Build history of the part. All positions in model axes, mm. Face numbers are marked on the shaded views. A direction names the side the tool comes from. Give positions to 0.01 mm unless a question says otherwise; leave off trailing zeros. Write each loop counter-clockwise with the first axis right and the second up, starting at its lowest first coordinate (ties: lowest second). Pieces come first, ordered by that corner, then holes. Notation, with made-up numbers: M -33.75,40.5 L -5.75,40.5 A21 cw -5.75,47.5 Z; hole C 2,32.25 d11. An arc over 180 degrees is marked long. One line per item, written item: value. Start each with the question number.
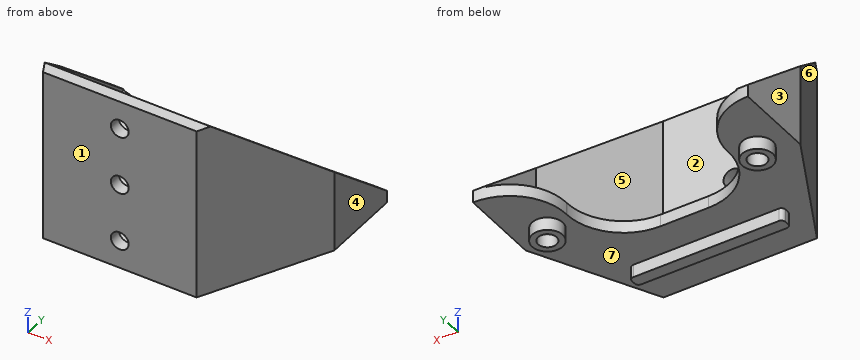
from build123d import *

# Parameters (mm, degrees)
F4_DEPTH       = 21.4
F5_DEPTH       = 1.5
F1_R           = 1.9
F1_W           = 19
F1_H           = 1.5
F6_DEPTH       = 1.6
F8_DEPTH       = 17.001
F8_DEPTH_BACK  = 17.001
F9_R           = 1.15
F10_DEPTH      = 21.401
F10_DEPTH_BACK = 1.601
F11_R          = 1.1
F12_DEPTH      = 1.5
F13_T1_DEPTH   = 1.5
F13_T3_DEPTH   = 36.5
F14_R          = 0.5


# Not quite as in the source:
# - a fillet or chamfer that OpenCascade refuses, or shapes differently, is made with other operations: its cross-section is extruded or revolved along the edge and cut away or added


with BuildPart() as f4:
    # F3 (on face) → F4 (new body)
    with BuildSketch(Plane.XY):
        Polygon((-15.5, 10), (-17, 10), (-17, 0), (-9.5, -14.7), (0, -14.7), (9.5, -14.7), (17, 0), (17, 10), (15.5, 10), (15.5, 0.3605454095), (8.5813543829, -13.2), (0, -13.2), (-8.5813543829, -13.2), (-15.5, 0.3605454095), align=None)
    extrude(amount=F4_DEPTH)

    # F2 (on Top) → F5 (join)
    with BuildSketch(Plane.XY):
        Polygon((-17, 0), (-9.5, -14.7), (0, -14.7), (9.5, -14.7), (17, 0), (17, 10), (10, 10), (10, -4.1), (0, -4.1), (-10, -4.1), (-10, 10), (-17, 10), align=None)
    extrude(amount=F5_DEPTH)

    # F1 (on Top) → F6 (join)
    with BuildSketch(Plane.XY):
        with Locations((-13, 2)):
            Circle(F1_R)
        with Locations((13, 2)):
            Circle(F1_R)
        with Locations((0, -8.95)):
            Rectangle(F1_W, F1_H)
    extrude(amount=-F6_DEPTH)

    # F7 (on Right) → F8 (cut, two sides)
    with BuildSketch(Plane.YZ) as f8_sk:
        Polygon((-13.2, 21.4), (10, 1.5), (10, 21.4), align=None)
    extrude(amount=-F8_DEPTH, mode=Mode.SUBTRACT)
    extrude(f8_sk.sketch, amount=F8_DEPTH_BACK, mode=Mode.SUBTRACT)

    # F9 (on Top) → F10 (cut, two sides)
    with BuildSketch(Plane.XY) as f10_sk:
        with Locations((13, 2)):
            Circle(F9_R)
        with Locations((-13, 2)):
            Circle(F9_R)
    extrude(amount=F10_DEPTH, mode=Mode.SUBTRACT)
    extrude(f10_sk.sketch, amount=-F10_DEPTH_BACK, mode=Mode.SUBTRACT)

    # F11 (on face) → F12 (cut, through all)
    with BuildSketch(Plane.XZ.offset(14.7)):
        with Locations((0, 3.475)):
            Circle(F11_R)
        with Locations((0, 17.925)):
            Circle(F11_R)
        with Locations((0, 10.7)):
            Circle(F11_R)
    extrude(amount=-F12_DEPTH, mode=Mode.SUBTRACT)

    # F13: fillet of radius 7 on 4 edges, made by hand

    # F13_s2 → F13_t1 (join)
    with BuildSketch(Plane.XY):
        with BuildLine():
            ThreePointArc((3, -4.1), (7.9497474683, -2.0497474683), (10, 2.9))
            Line((10, 2.9), (10, -4.1))
            Line((10, -4.1), (3, -4.1))
        make_face()
        with BuildLine():
            ThreePointArc((-10, 2.9), (-7.9497474683, -2.0497474683), (-3, -4.1))
            Line((-3, -4.1), (-10, -4.1))
            Line((-10, -4.1), (-10, 2.9))
        make_face()
    extrude(amount=F13_T1_DEPTH)

    # F13_s4 → F13_t3 (cut)
    with BuildSketch(Plane.XY.offset(-17.5)):
        with BuildLine():
            ThreePointArc((-17, 10), (-12.0502525317, 7.9497474683), (-10, 3))
            Line((-10, 3), (-10, 10))
            Line((-10, 10), (-17, 10))
        make_face()
        with BuildLine():
            ThreePointArc((10, 3), (12.0502525317, 7.9497474683), (17, 10))
            Line((17, 10), (10, 10))
            Line((10, 10), (10, 3))
        make_face()
    extrude(amount=F13_T3_DEPTH, mode=Mode.SUBTRACT)

    # F14
    f14_edges = [f4.edges().sort_by_distance(p)[0] for p in [
        (-9.5, -8.2, -0.8),
        (-9.5, -9.7, -0.8),
        (9.5, -8.2, -0.8),
        (9.5, -9.7, -0.8),
    ]]
    fillet(f14_edges, radius=F14_R)


solid = f4.part
1) Band-saw the part on B-B (x = 0). List the corners of the cut face in (y, z) (3 decimals), then the cut area to 4 significant figures.
2) Drop flat-ended pins along their axis: P1, Ø1.3, axis at x = 0, z = 3.475, coming from the -Y side; P2, Ø5, axis at y = -12, z = 2, coming from the +X side; P3, Ø2.5, axis at x = -13, y = 2, coming from the +Z side; P4, Ø3.5, axis at x = 0, z = 10.7, coming from the +Y side. Give the stop position or say it passes through.
3) Tool access for the marked faces 5, 6 and 7: list every direction of +Z, -Z, +X, -X, +Y, -Y with a clear straight run to the whole face (end or side of a thin tool).
4) Band-saw the part on A-A (z = 1). List the corners of the cut face in (x, y).
5) Band-saw the part on D-D (z = 10.7). List the corners of the cut face in (x, y), then the cut area to 3 significant figures.
6) Band-saw the part on C-C (y = 5.5). List the corners of the cut face in (x, z), then the cut area to 3 significant figures.
7) Mould opens along X. For the marked faces 1, 2, 3 and 4 say: released by +X, released by -X, zero draft, split by the parting line, or undercut.
8) Probe line 1 along Z through (x, y) = (0, -14.3) (3 decimals); line 2 along X through (y, z) = (2, 1.2); line 3 along Y through (x, z) = (-13, -1.05). List the from-to ranges inside material, lowest first. Write a range as from..to.
Model answer:
1. outline: M -14.7,0 L -9.7,0 L -9.7,-1.6 L -8.2,-1.6 L -8.2,0 L -4.1,0 L -4.1,1.5 L -13.2,1.5 L -13.2,2.375 L -14.7,2.375 Z; M -14.7,4.575 L -13.2,4.575 L -13.2,9.6 L -14.7,9.6 Z; M -14.7,11.8 L -13.2,11.8 L -13.2,16.825 L -14.7,16.825 Z; M -14.7,19.025 L -13.2,19.025 L -13.2,21.4 L -14.7,21.4 Z
1. area: 38.25 mm²
2. P1: passes through
2. P2: stops at x = 12.15
2. P3: stops at z = 1.5
2. P4: stops at y = -13.2
3. face 5: +Z, +Y
3. face 6: +Z, -Z, -X, -Y
3. face 7: -Z
4. outline: M -17,0 L -9.5,-14.7 L 9.5,-14.7 L 17,0 L 17,10 A7 ccw 10,3 L 10,2.9 A7 cw 3,-4.1 L -3,-4.1 A7 cw -10,2.9 L -10,3 A7 ccw -17,10 Z; hole C -13,2 d2.3; hole C 13,2 d2.3
5. outline: M -16.63,-0.73 L -9.5,-14.7 L -1.1,-14.7 L -1.1,-13.2 L -8.58,-13.2 L -14.95,-0.73 Z; M 1.1,-14.7 L 9.5,-14.7 L 16.63,-0.73 L 14.95,-0.73 L 8.58,-13.2 L 1.1,-13.2 Z
5. area: 68.4 mm²
6. outline: M -17,0 L -10.46,0 L -10.46,1.5 L -15.5,1.5 L -15.5,5.36 L -17,5.36 Z; M 10.46,0 L 17,0 L 17,5.36 L 15.5,5.36 L 15.5,1.5 L 10.46,1.5 Z
6. area: 31.2 mm²
7. face 1: zero draft
7. face 2: undercut
7. face 3: released by -X
7. face 4: released by +X
8. line 1: z = 0..2.375, 4.575..9.6, 11.8..16.825, 19.025..21.4
8. line 2: x = -17..-14.15, -11.85..-9.94, 9.94..11.85, 14.15..17
8. line 3: y = 0.1..0.85, 3.15..3.9
